Could you check a few things on this model? Use its own coordinates, in mm. A direction names the side the tool comes from. Round coordinates to 2 decimals unless told otherwise and drop trailing zeros. Order: outer loops, then holes, each group sorted by start corner. A loop starts at its lowest first (then second) coordinate and runs counter-clockwise, first axis right, second up. Notation, with made-up numbers: (70.25, 70) -> (85.25, 70) arc R21 cw to (85.25, 91) -> close; hole circle Ø8 at (33.25, 19). An arc over 180 degrees is marked (long way). One line per question, with ' | ' between items.
Autodesk Inventor part; units mm, degrees
ref_plane "YZ Plane" through (0, 0, 0) normal (1, 0, 0) x (0, 1, 0)
ref_plane "XZ Plane" through (0, 0, 0) normal (0, 1, 0) x (-1, 0, 0)
ref_plane "XY Plane" through (0, 0, 0) normal (0, 0, 1) x (1, 0, 0)
sketch "스케치1" plane through (0, 0, 0) normal (0, 0, 1) x (1, 0, 0)
  line L0 (0, 0) -> (150, 0)
  line L1 (150, 0) -> (150, 150)
  line L2 (0, 150) -> (0, 0)
  line L3 (0, 80) -> (150, 80)
  line L4 (0, 5) -> (150, 5)
  line L5 (0, 150) -> (10, 150)
  line L6 (10, 150) -> (10, 80)
  line L7 (10, 80) -> (0, 80)
  line L8 (0, 80) -> (0, 150)
  line L9 (150, 150) -> (140, 150)
  line L10 (140, 150) -> (140, 80)
  line L11 (140, 80) -> (150, 80)
  line L12 (150, 80) -> (150, 150)
  line L13 (150, 150) -> (140, 150)
  line L14 (10, 150) -> (0, 150)
  dimension "d0" = 150
  dimension "d1" = 150
  dimension "d2" = 80
  dimension "d3" = 5
  dimension "d4" = 10
  dimension "d5" = 10
extrude "돌출1" add sketch "스케치1" along normal blind 150 contours L2 L4 L1 L0
extrude "돌출2" add sketch "스케치1" along normal blind 5 contours L2 L3 L1 L4
extrude "돌출3" add sketch "스케치1" along normal blind 5 contours L2 L5 L6 L3 | L3 L10 L9 L1
sketch "스케치2" plane through (0, 5, 150) normal (0, 1, 0) x (1, 0, 0)
  line L0 (150, 145) -> (0, 145)
  line L1 (0, 145) -> (0, 0)
  line L2 (150, 0) -> (0, 0)
  line L3 (150, 145) -> (150, 0)
  line L4 (140, 145) -> (140, 150)
  line L5 (140, 150) -> (10, 150)
  line L6 (10, 150) -> (10, 145)
  line L7 (140, 145) -> (10, 145)
  line L8 (10, 150) -> (0, 150)
  line L9 (0, 150) -> (0, 145)
  line L10 (10, 145) -> (0, 145)
  line L11 (10, 150) -> (10, 145)
  line L12 (150, 150) -> (140, 150)
  line L13 (140, 150) -> (140, 145)
  line L14 (150, 145) -> (140, 145)
  line L15 (150, 150) -> (150, 145)
  line L16 (0, 150) -> (5, 150)
  line L17 (5, 150) -> (5, 140)
  line L18 (5, 140) -> (0, 140)
  line L19 (0, 140) -> (0, 150)
  line L20 (0, 150) -> (150, 150)
  line L21 (0, 150) -> (0, 140)
  line L22 (5, 140) -> (5, 145)
  line L23 (10, 145) -> (10, 150)
  line L24 (0, 75) -> (150, 75)
  line L25 (150, 145) -> (150, 0)
  line L26 (75, 0) -> (75, 150)
  line L27 (10, 0) -> (10, 5)
  line L28 (10, 0) -> (0, 0)
  line L29 (5, 5) -> (5, 10)
  line L30 (5, 10) -> (0, 10)
  line L31 (0, 10) -> (0, 0)
  line L32 (5, 5) -> (10, 5)
  line L33 (5, 145) -> (10, 145)
  line L34 (10, 150.1761) -> (0, 150)
  line L35 (10, 0) -> (0, 0)
  line L36 (0, 145) -> (150, 145)
  line L37 (150, 145) -> (150, 0)
  line L38 (0, 0) -> (150, 0)
  line L39 (140, 150) -> (140, 145)
  line L40 (145, 140) -> (150, 140)
  line L41 (145, 140) -> (145, 145)
  line L42 (145, 10) -> (150, 10)
  line L43 (150, 10) -> (150, 0)
  line L44 (145, 5) -> (145, 10)
  line L45 (145, 5) -> (140, 5)
  line L46 (140, 0) -> (140, 5)
  point P0 (5, 0)
  point P1 (140, 5)
  point P2 (140, 0)
  point P3 (150, 10)
  point P4 (0, 10)
  point P5 (0, 140)
  dimension "d12" = 5
  dimension "d13" = 10
  dimension "d14" = 150
  dimension "d15" = 10
  dimension "d16" = 150
  dimension "d17" = 150
extrude "돌출4" add sketch "스케치2" along normal blind 145 contours L3 L40 L41 L0 | L3 L2 L46 L45 L44 L42 | L17 L18 L1 L0 | L30 L29 L32 L27 L2 L1
properties part number "적재부 하판"
1. I'm going to push flat-ended pins straight in: pin 1 (4 mm diameter, centred on x = 32.5, z = 57.5, fed in from +Y); pin 2 (4 mm diameter, centred on x = 102, z = 1.5, fed in from +Y). Where does each tip first touch, or does it pass through?
From the geometry:
pin 1: stops at y = 5 | pin 2: stops at y = 80
2. I want a section at A-A on y = 123.5. List the corners of the cut face in (x, z) for me, and give its area (3 significant figures).
From the geometry:
outline: (0, 0) -> (10, 0) -> (10, 5) -> (5, 5) -> (5, 10) -> (0, 10) -> close; (0, 140) -> (5, 140) -> (5, 145) -> (10, 145) -> (10, 150) -> (0, 150) -> close; (140, 0) -> (150, 0) -> (150, 10) -> (145, 10) -> (145, 5) -> (140, 5) -> close; (140, 145) -> (145, 145) -> (145, 140) -> (150, 140) -> (150, 150) -> (140, 150) -> close | area: 300 mm²
3. I want a section at B-B on y = 52. List the corners of the cut face in (x, z) for me, and give its area (3 significant figures).
From the geometry:
outline: (0, 0) -> (150, 0) -> (150, 10) -> (145, 10) -> (145, 5) -> (5, 5) -> (5, 10) -> (0, 10) -> close; (0, 140) -> (5, 140) -> (5, 145) -> (10, 145) -> (10, 150) -> (0, 150) -> close; (140, 145) -> (145, 145) -> (145, 140) -> (150, 140) -> (150, 150) -> (140, 150) -> close | area: 950 mm²
4. On a 3-axis mill with a long thin cutter (end or side, diameter ignored), from which of +Z, -Z, +X, -X, +Y, -Y can I reach the whole of each face in a straight line? I mean faces 1 (the face through (5, 76, 7)), 2 (the face through (10, 76, 148)), 3 (the face through (146, 150, 146)), 4 (the face through (10, 115, 2)), 5 (the face through (147, 76, 10)). Say none if no direction works.
From the geometry:
face 1: +Y | face 2: +Z, +Y | face 3: +Z, -Z, +X, -X, +Y | face 4: +Z, -Z, +Y | face 5: +X, -X, +Y
5. I need wall thicknesses on probe 1 along Z at (x, y) = (9, 11); probe 2 along Y at (x, z) = (30.5, 27.5). Which ranges of each line are inside material? Lowest first, please.
From the geometry:
probe 1: z = 0 to 5, 145 to 150 | probe 2: y = 0 to 5
6. If we mould it in two halves opening along Z, with no side actions, what happens to faces 6 (the face through (3, 76, 140)), 7 (the face through (75, 3, 150)), 8 (the face through (74, 80, 2))? For each: pulls with the +Z half, pulls with the -Z half, needs draft (parallel to the pull), parting line crosses it, or undercut.
From the geometry:
face 6: undercut | face 7: pulls with the +Z half | face 8: needs draft
7. I want a section at D-D on z = 37.5. List the corners of the cut face in (x, y) for me, and give its area (3 significant figures).
From the geometry:
outline: (0, 0) -> (150, 0) -> (150, 5) -> (0, 5) -> close | area: 750 mm²
8. I want a section at C-C on x = 135. List the corners of the cut face in (y, z) for me.
From the geometry:
outline: (0, 0) -> (80, 0) -> (80, 5) -> (5, 5) -> (5, 150) -> (0, 150) -> close
